Geometry: see drawing. Coordinates: mm, zero at the bounding-box minimum. A direction names the side the tool comes from. Coordinates: 2 decimals unless noted, no trailing zeros. Order: outer loops, then holes, each group sorted by start corner. A loop starts at its lowest first (then second) coordinate and runs counter-clockwise, first axis right, second up. Notation, with made-up numbers: M 33.5,-14 L 89.5,-14 A21 cw 89.5,4 Z; hole C 75,44 d5. An arc over 180 degrees is marked long. Answer in a Markdown table with one row per item.
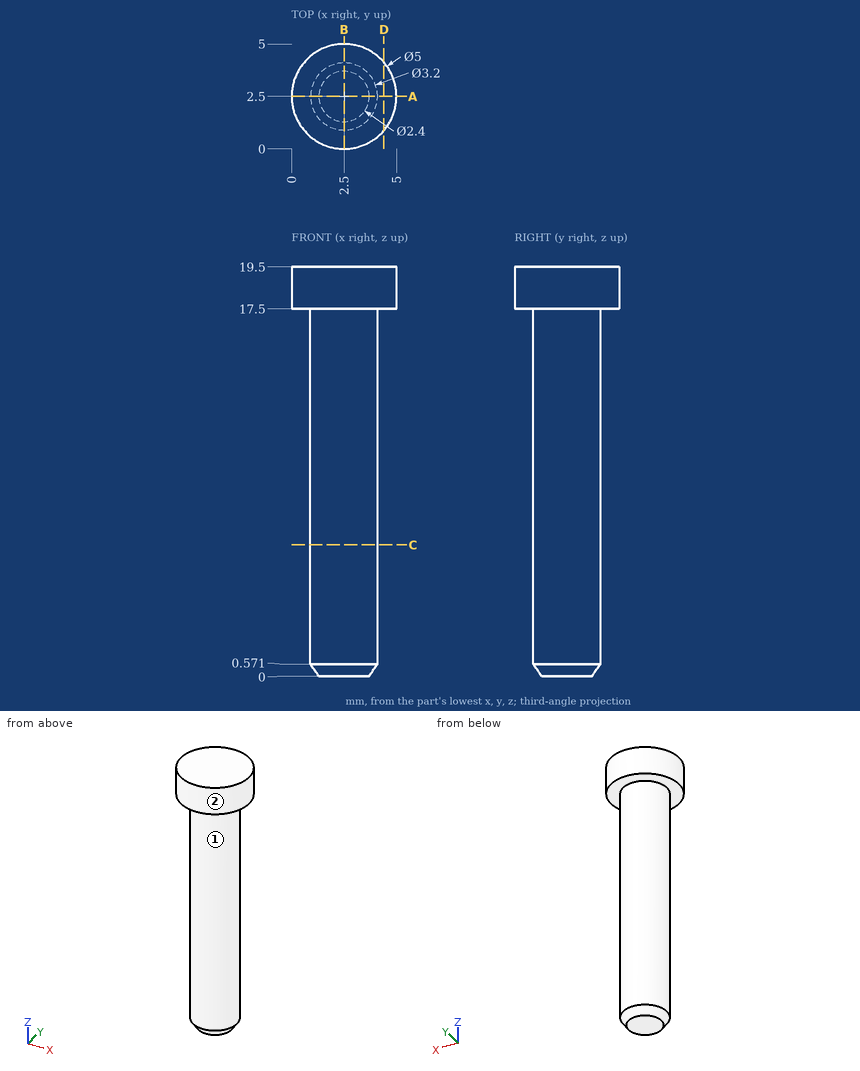
1) Cut plane D-D, the plane x = 4.4. Output: boundary loops of the cut face in (y, z) (1 decimal).
Resolved:
| item | result |
|---|---|
| outline | M 0.9,17.5 L 4.1,17.5 L 4.1,19.5 L 0.9,19.5 Z |
2) Cut plane C-C, the plane z = 6.25. Output: boundary loops of the cut face in (x, y).
Resolved:
| item | result |
|---|---|
| outline | C 2.5,2.5 d3.2 |
3) Material intervals for probe 1 along Z at (x, y) = (4.4, 3.5); probe 2 along X at (y, z) = (2.35, 2.5); probe 3 along Z at (x, y) = (2.75, 0.95), sorted ascending.
Resolved:
| item | result |
|---|---|
| probe 1 | z = 17.5 to 19.5 |
| probe 2 | x = 0.91 to 4.09 |
| probe 3 | z = 0.53 to 19.5 |
4) Reachability of the marked faces 1 and 2 from +Z, -Z, +X, -X, +Y, -Y: full face, straight path, thin tool, end or side. Return the list, or none.
Resolved:
| item | result |
|---|---|
| face 1 | -Z |
| face 2 | +Z, -Z |
5) Contact query for flat-ended pins moving along their axis: pin 1 (1.5 mm diameter, centred on y = 4.5, z = 11.5, fed in from +X); pin 2 (1.5 mm diameter, centred on y = 1, z = 2.5, fed in from -X); pin 3 (1.5 mm diameter, centred on y = 2.5, z = 9, fed in from -X). Output: stop coordinate, or through.
Resolved:
| item | result |
|---|---|
| pin 1 | stops at x = 3.5 |
| pin 2 | stops at x = 1.09 |
| pin 3 | stops at x = 0.9 |
6) Cut plane A-A, the plane y = 2.5. Output: boundary loops of the cut face in (x, z).
Resolved:
| item | result |
|---|---|
| outline | M 0,17.5 L 0.9,17.5 L 0.9,0.57 L 1.3,0 L 3.7,0 L 4.1,0.57 L 4.1,17.5 L 5,17.5 L 5,19.5 L 0,19.5 Z |
